from build123d import *

# Parameters (mm, degrees)
ESQUISSE1_R        = 2.25
ESQUISSE1_R_2      = 3
BOSS_EXTRU_1_DEPTH = 1


with BuildPart() as part:
    # Esquisse1 → Boss.-Extru.1 (new, symmetric)
    with BuildSketch(Plane.XY):
        with BuildLine():
            Line((21, 31.5), (146, 31.5))
            ThreePointArc((146, 31.5), (156, 21.5), (146, 11.5))
            Line((146, 11.5), (33.5, 11.5))
            ThreePointArc((33.5, 11.5), (25, 3), (33.5, -5.5))
            Line((33.5, -5.5), (35.75, -5.5))
            ThreePointArc((35.75, -5.5), (40, -9.75), (35.75, -14))
            Line((35.75, -14), (27, -14))
            ThreePointArc((27, -14), (11.214469473, -16.988397735), (-4.686322253, -14.690938802))
            ThreePointArc((-4.686322253, -14.690938802), (-13.539380352, -7.380411831), (-14.886645987, 4.02157561))
            ThreePointArc((-14.886645987, 4.02157561), (-1.599309542, 23.841476371), (21, 31.5))
        make_face()
        with Locations((35.75, -9.75)):
            Circle(ESQUISSE1_R, mode=Mode.SUBTRACT)
        Circle(ESQUISSE1_R_2, mode=Mode.SUBTRACT)
        with BuildLine():
            Line((15, 23.5), (39, 23.5))
            ThreePointArc((39, 23.5), (41, 21.5), (39, 19.5))
            Line((39, 19.5), (15, 19.5))
            ThreePointArc((15, 19.5), (13, 21.5), (15, 23.5))
        make_face(mode=Mode.SUBTRACT)
        with BuildLine():
            Line((48, 23.5), (113, 23.5))
            ThreePointArc((113, 23.5), (115, 21.5), (113, 19.5))
            Line((113, 19.5), (48, 19.5))
            ThreePointArc((48, 19.5), (46, 21.5), (48, 23.5))
        make_face(mode=Mode.SUBTRACT)
        with BuildLine():
            Line((122, 23.5), (146, 23.5))
            ThreePointArc((146, 23.5), (148, 21.5), (146, 19.5))
            Line((146, 19.5), (122, 19.5))
            ThreePointArc((122, 19.5), (120, 21.5), (122, 23.5))
        make_face(mode=Mode.SUBTRACT)
        with BuildLine():
            ThreePointArc((13.266499161, -7), (12.845232579, 7.745966692), (0, 15))
            ThreePointArc((0, 15), (-2, 13), (0, 11))
            ThreePointArc((0, 11), (9.419837224, 5.680375574), (9.728766052, -5.133333333))
            ThreePointArc((9.728766052, -5.133333333), (10.564299273, -7.835533222), (13.266499161, -7))
        make_face(mode=Mode.SUBTRACT)
    extrude(amount=BOSS_EXTRU_1_DEPTH, both=True)


solid = part.part
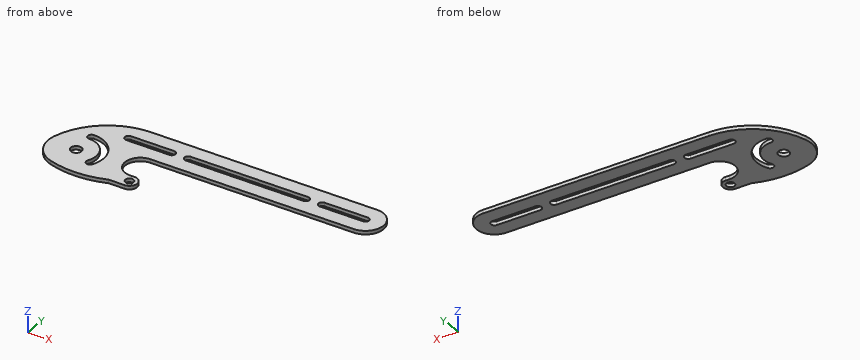
Could you check a few things on this model? Use its own coordinates, in mm. Give positions to 0.01 mm unless a question says otherwise; leave off trailing zeros. Order: outer loops, then holes, each group sorted by start corner. A loop starts at its lowest first (then second) coordinate and runs counter-clockwise, first axis right, second up. Notation, with made-up numbers: (45.5, 48.25) -> (63.5, 48.25) arc R38 cw to (63.5, 86.25) -> close; hole circle Ø3 at (-6, 1). An arc over 180 degrees is marked (long way). Answer in a Markdown table with one row per item. Add a question column.
Item 1: Imagine slicing it at A-A (x = 76). List the corners of the cut face in (y, z) for me.
Item 2: Imagine slicing it at C-C (z = 0.55). List the corners of the cut face in (x, y) for me.
Item 3: Imagine slicing it at B-B (y = 9.5). List the corners of the cut face in (x, z) for me.
Item 4: Please list where these lines run through material, in increasing order: probe 1 along Y at (x, z) = (35.75, -0.35); probe 2 along Y at (x, z) = (139, 0.05); probe 3 along Y at (x, z) = (2, -0.4).
Item 5: I'm going to push flat-ended pins straight in: P1, Ø1, axis at y = 13.5, z = 0, coming from the +X side; P2, Ø1, axis at x = 68.5, z = 0, coming from the -Y side; P3, Ø0.6, axis at x = 33, z = 0, coming from the -Y side. Where does each tip first touch, or does it pass through?
Result:
| question | item | result |
|---|---|---|
| 1 | outline | (11.5, -1) -> (19.5, -1) -> (19.5, 1) -> (11.5, 1) -> close; (23.5, -1) -> (31.5, -1) -> (31.5, 1) -> (23.5, 1) -> close |
| 2 | outline | (-14.89, 4.02) arc R15.42 ccw to (-4.69, -14.69) arc R48.82 ccw to (27, -14) -> (35.75, -14) arc R4.25 ccw to (35.75, -5.5) -> (33.5, -5.5) arc R8.5 cw to (33.5, 11.5) -> (146, 11.5) arc R10 ccw to (146, 31.5) -> (21, 31.5) arc R37.17 ccw to start; hole circle Ø6 at (0, 0); hole (0, 11) arc R11 cw to (9.73, -5.13) arc R2 ccw to (13.27, -7) arc R15 ccw to (0, 15) arc R2 ccw to start; hole (15, 19.5) -> (39, 19.5) arc R2 ccw to (39, 23.5) -> (15, 23.5) arc R2 ccw to start; hole circle Ø4.5 at (35.75, -9.75); hole (48, 19.5) -> (113, 19.5) arc R2 ccw to (113, 23.5) -> (48, 23.5) arc R2 ccw to start; hole (122, 19.5) -> (146, 19.5) arc R2 ccw to (146, 23.5) -> (122, 23.5) arc R2 ccw to start |
| 3 | outline | (-12.94, -1) -> (5.55, -1) -> (5.55, 1) -> (-12.94, 1) -> close; (11.61, -1) -> (28.02, -1) -> (28.02, 1) -> (11.61, 1) -> close |
| 4 | probe 1 | -14 to -12, -7.5 to -5.5, 11.5 to 19.5, 23.5 to 31.5 |
| 4 | probe 2 | 11.5 to 19.5, 23.5 to 31.5 |
| 4 | probe 3 | -16.31 to -2.24, 2.24 to 10.82, 14.87 to 26.28 |
| 5 | P1 | x = 152.61 |
| 5 | P2 | y = 11.5 |
| 5 | P3 | y = -14 |
